```python
from build123d import *

# Parameters (mm, degrees)
SKETCH_1_W          = 30
SKETCH_1_H          = 185
EXTRUDE_1_DEPTH     = 5
SKETCH_2_R          = 6
SKETCH_2_R_2        = 3
CUT_EXTRUDE_1_DEPTH = 94.841621896
FILLET_1_R          = 10
SKETCH_5_W          = 35
SKETCH_5_H          = 30
EXTRUDE_3_DEPTH     = 5
FILLET_4_R          = 10
FILLET_5_R          = 18
CUT_EXTRUDE_3_DEPTH = 5
CUT_EXTRUDE_4_DEPTH = 5
EXTRUDE_START       = -5
EXTRUDE_5_DEPTH     = 5
SKETCH_11_R         = 1.5
CUT_EXTRUDE_5_DEPTH = 106.267516357
SKETCH_12_R         = 9
SKETCH_12_R_2       = 7.5
CUT_EXTRUDE_6_DEPTH = 106.267516357
CUT_EXTRUDE_7_DEPTH = 106.267516357
FILLET_9_R          = 5
FILLET_10_R         = 3
FILLET_11_R         = 5
FILLET_12_R         = 20


with BuildPart() as part:
    # 草图1 → 凸台-拉伸1 (new body)
    with BuildSketch(Plane.XY):
        Rectangle(SKETCH_1_W, SKETCH_1_H)
    extrude(amount=EXTRUDE_1_DEPTH)

    # 草图2 → 切除-拉伸1 (cut, through all)
    with BuildSketch(Plane.XY.offset(5)):
        with Locations((0, 80.5)):
            Circle(SKETCH_2_R)
        with Locations((0, -82.5)):
            Circle(SKETCH_2_R_2)
    extrude(amount=-CUT_EXTRUDE_1_DEPTH, mode=Mode.SUBTRACT)

    # 圆角1
    fillet_1_edges = [part.edges().sort_by_distance(p)[0] for p in [
        (-15, 92.5, 2.5),
        (15, 92.5, 2.5),
    ]]
    fillet(fillet_1_edges, radius=FILLET_1_R)

    # 草图5 → 凸台-拉伸3 (add)
    with BuildSketch(Plane.XY.offset(5)):
        with Locations((32.5, 52.5)):
            Rectangle(SKETCH_5_W, SKETCH_5_H)
    extrude(amount=-EXTRUDE_3_DEPTH)

    # 圆角4
    fillet_4_edges = [part.edges().sort_by_distance(p)[0] for p in [
        (15, 37.5, 2.5),
        (15, 67.5, 2.5),
        (50, 67.5, 2.5),
        (50, 37.5, 2.5),
    ]]
    fillet(fillet_4_edges, radius=FILLET_4_R)

    # 圆角5
    # the kernel refuses this fillet: 18 mm, written as the material it takes off along each edge
    with BuildSketch(Plane(origin=(-15, -92.5, -45), x_dir=(0, 1, 0), z_dir=(0, 0, 1)), Plane(origin=(15, -92.5, -45), x_dir=(-1, 0, 0), z_dir=(0, 0, 1))) as fillet_5_piece_1:
        with BuildLine():
            CenterArc((FILLET_5_R, -FILLET_5_R), FILLET_5_R, 90, 90)
            Line((0, -FILLET_5_R), (0, 0))
            Line((0, 0), (FILLET_5_R, 0))
        make_face()
    extrude(amount=95, mode=Mode.SUBTRACT)

    # 草图8 → 切除-拉伸3 (cut)
    with BuildSketch(Plane(origin=(0, 0, 0), x_dir=(-1, 0, 0), z_dir=(0, 0, -1))):
        with BuildLine():
            Line((-4.1, 60.5), (-4.1, -7.5))
            ThreePointArc((-4.1, -7.5), (0, -11.6), (4.1, -7.5))
            Line((4.1, -7.5), (4.1, 60.5))
            ThreePointArc((4.1, 60.5), (0, 64.6), (-4.1, 60.5))
        make_face()
    extrude(amount=-CUT_EXTRUDE_3_DEPTH, mode=Mode.SUBTRACT)

    # 草图9 → 切除-拉伸4 (cut)
    with BuildSketch(Plane.XY.offset(5)):
        Polygon((22.949354722, 80.050183125), (35, 61.5), (47.495924497, 69.617653207), align=None)
    extrude(amount=-CUT_EXTRUDE_4_DEPTH, mode=Mode.SUBTRACT)

    # 草图10 → 凸台-拉伸5 (add)
    with BuildSketch(Plane.XY.offset(5).offset(EXTRUDE_START)):
        with BuildLine():
            Line((25, 37.5), (40, 37.5))
            ThreePointArc((40, 37.5), (46.005154783, 39.503868684), (49.603601244, 44.712376794))
            Line((49.603601244, 44.712376794), (15, -74.5))
            Line((15, -74.5), (15, 27.5))
            ThreePointArc((15, 27.5), (17.928932188, 34.571067812), (25, 37.5))
        make_face()
    extrude(amount=EXTRUDE_5_DEPTH)

    # 草图11 → 切除-拉伸5 (cut, through all)
    with BuildSketch(Plane.XY.offset(5)):
        with Locations((-7, -22.5)):
            Circle(SKETCH_11_R)
        with Locations((17.544259481, -27.251770883)):
            Circle(SKETCH_11_R)
        with Locations((18.828850642, -7.5)):
            Circle(SKETCH_11_R)
        with Locations((28.585531862, 26.112604356)):
            Circle(SKETCH_11_R)
        with Locations((30, 50.5)):
            Circle(SKETCH_11_R)
        with Locations((-9, 2.5)):
            Circle(SKETCH_11_R)
    extrude(amount=-CUT_EXTRUDE_5_DEPTH, mode=Mode.SUBTRACT)

    # 草图12 → 切除-拉伸6 (cut, through all)
    with BuildSketch(Plane.XY.offset(5)):
        with Locations((20, 42.5)):
            Circle(SKETCH_12_R)
        with Locations((20, -2.5)):
            Circle(SKETCH_12_R_2)
        with Locations((3, -37.5)):
            Circle(SKETCH_12_R)
        with Locations((3, -62.5)):
            Circle(SKETCH_12_R_2)
    extrude(amount=-CUT_EXTRUDE_6_DEPTH, mode=Mode.SUBTRACT)

    # 草图13 → 切除-拉伸7 (cut, through all)
    with BuildSketch(Plane.XY.offset(5)):
        Polygon((22.804344395, 76.602108744), (34.957124842, 57.894703657), (54.492950931, 70.585646319), align=None)
    extrude(amount=-CUT_EXTRUDE_7_DEPTH, mode=Mode.SUBTRACT)

    # 圆角9
    fillet_9_edges = [part.edges().sort_by_distance(p)[0] for p in [
        (46.30180901, 65.264483447, 2.5),
        (28.717293233, 67.5, 2.5),
    ]]
    fillet(fillet_9_edges, radius=FILLET_9_R)

    # 圆角10
    fillet_10_edges = [part.edges().sort_by_distance(p)[0] for p in [
        (34.957124842, 57.894703657, 2.5),
    ]]
    fillet(fillet_10_edges, radius=FILLET_10_R)

    # 圆角11
    fillet_11_edges = [part.edges().sort_by_distance(p)[0] for p in [
        (0, -92.248239349, 2.5),
    ]]
    fillet(fillet_11_edges, radius=FILLET_11_R)

    # 圆角12
    fillet_12_edges = [part.edges().sort_by_distance(p)[0] for p in [
        (15, -74.5, 2.5),
    ]]
    fillet(fillet_12_edges, radius=FILLET_12_R)


solid = part.part
```
Can you work these out from the model? Positions are in its coordinate system, mm. A direction names the side the tool comes from. Coordinates: 2 decimals unless noted, no trailing zeros. Write each loop counter-clockwise with the first axis right and the second up, starting at its lowest first coordinate (ties: lowest second). Pieces come first, ordered by that corner, then holes. Notation, with made-up numbers: (54, 80.5) - (76, 80.5) arc R20 ccw to (76, 117.5) - close; hole circle Ø4 at (77, 58.5). An arc over 180 degrees is marked (long way). Return JSON: item names as keys, results as strings.
Q1. If we section it at A-A (y = 80.5): Please give me the cut outline in (x, z), then the cut area to 3 significant figures.
Computed values:
{"outline": "(-15, 0) - (-6, 0) - (-6, 5) - (-15, 5) - close; (6, 0) - (15, 0) - (15, 5) - (6, 5) - close", "area": "90.0 mm2"}
Q2. Thinking about a two-plate mould opening in X: for faces 1 (the flat face through (32.862, -12.965, 2.465)), 2 (the cylindrical face through (16.046, -27.186, 2.535)), 3 (the flat face through (11, 1, 5)), which applies, +X half, -X half, draft (parallel to the pull), parting line (faces both ways), or undercut?
Computed values:
{"face 1": "+X half", "face 2": "undercut", "face 3": "draft"}
Q3. On a 3-axis mill with a long thin cutter (end or side, diameter ignored), from which of +Z, -Z, +X, -X, +Y, -Y can I reach the whole of each face in a straight line? I mean faces 4 (the flat face through (-4.1, 26, 2)), 5 (the cylindrical face through (10.51, -86.395, 2.465)), 6 (the flat face through (50, 52, 3)), 7 (the flat face through (15, 80, 2)), 8 (the flat face through (39.8, 61.04, 2.54)). Say none if no direction works.
Computed values:
{"face 4": "+Z, -Z", "face 5": "+Z, -Z, +X, -Y", "face 6": "+Z, -Z, +X, +Y, -Y", "face 7": "+Z, -Z, +X, +Y", "face 8": "+Z, -Z, +Y"}
Q4. If we section it at C-C (y = 42.5): Please give me the cut outline in (x, z), then the cut area to 3 significant figures.
Computed values:
{"outline": "(-15, 0) - (-4.1, 0) - (-4.1, 5) - (-15, 5) - close; (4.1, 0) - (11, 0) - (11, 5) - (4.1, 5) - close; (29, 0) - (48.96, 0) - (48.96, 5) - (29, 5) - close", "area": "189 mm2"}
Q5. If we section it at B-B (x = 8.5): Please give me the cut outline in (y, z).
Computed values:
{"outline": "(-88.35, 0) - (-67.6, 0) - (-67.6, 5) - (-88.35, 5) - close; (-57.4, 0) - (-44.62, 0) - (-44.62, 5) - (-57.4, 5) - close; (-30.38, 0) - (91.87, 0) - (91.87, 5) - (-30.38, 5) - close"}
Q6. I'm going to push flat-ended pins straight in: pin 1 Ø1.5 at (y, z) = (79.5, 2) entering from +X; pin 2 Ø2.5 at (x, y) = (-7, -22.5) entering from -Z. Where does each tip first touch, or does it pass through?
Computed values:
{"pin 1": "stops at x = 15", "pin 2": "passes through"}
Q7. If we section it at D-D (y = 12): Please give me the cut outline in (x, z), then the cut area to 3 significant figures.
Computed values:
{"outline": "(-15, 0) - (-4.1, 0) - (-4.1, 5) - (-15, 5) - close; (4.1, 0) - (40.11, 0) - (40.11, 5) - (4.1, 5) - close", "area": "235 mm2"}
Q8. Please list where these lines run through material, in increasing order: L1, parallel to X at y = 48, z = 3.7; L2, parallel to Y at x = -3.5, z = 2.95; L3, parallel to X at y = 56, z = 3.8. Write a range as from..to.
Computed values:
{"L1": "x = -15..-4.1, 4.1..12.88, 27.12..50", "L2": "y = -91.29..-66.24, -58.76..-43.72, -31.28..-9.64, 62.64..75.63, 85.37..92.5", "L3": "x = -15..-4.1, 4.1..50"}
